Read the model definition and answer for the solid it produces. Units are mm, in the model's axes. Give positions to 0.01 mm unless a question says otherwise; leave off trailing zeros. Order: outer loops, then holes, each group sorted by start corner. A loop starts at its lowest first (then second) coordinate and runs counter-clockwise, first axis right, second up.
Item 1: A cutting plane is placed at A-A (x = -206.5). Write down the section's boundary in (y, z), plus the area to 3 significant figures.
Item 2: A cutting plane is placed at C-C (x = 59.5). Write down the section's boundary in (y, z).
Item 3: A cutting plane is placed at D-D (z = 1.45). State how many separate pieces and enclosed holes the cut face has, plus the area to 3 significant figures.
Item 4: A cutting plane is placed at B-B (y = 66.5). Write down the section's boundary in (x, z).
Item 5: Given pin 1 Ø1.5 at (x, z) = (198.5, 1) entering from -Y; pin 2 Ø0.9 at (y, z) = (233, 2) entering from -X; pin 3 Ø1.5 at (x, z) = (180, 2) entering from +Y, each flat-ended and moving along its own axis, determine where each tip first touches the part or whether it passes through.
Item 6: Find the intervals of material crossed by line 1 along X through (y, z) = (-255, 0.8); line 2 along X through (y, z) = (100, 1.2); line 3 along X through (y, z) = (-108, 1.1), in increasing order.
from build123d import *

# Parameters (mm, degrees)
EXTRUDE_1_DEPTH     = 3
SKETCH_2_R          = 1
CUT_EXTRUDE_1_DEPTH = 3


with BuildPart() as part:
    # 草图1 → 凸台-拉伸1 (new body)
    with BuildSketch(Plane.XY):
        with BuildLine():
            Line((-140, -280), (140, -280))
            ThreePointArc((140, -280), (147.071067812, -277.071067812), (150, -270))
            Line((150, -270), (150, -170))
            ThreePointArc((150, -170), (152.928932188, -162.928932188), (160, -160))
            Line((160, -160), (260, -160))
            ThreePointArc((260, -160), (267.071067812, -157.071067812), (270, -150))
            Line((270, -150), (270, 150))
            ThreePointArc((270, 150), (267.071067812, 157.071067812), (260, 160))
            Line((260, 160), (160, 160))
            ThreePointArc((160, 160), (152.928932188, 162.928932188), (150, 170))
            Line((150, 170), (150, 275))
            ThreePointArc((150, 275), (148.535533906, 278.535533906), (145, 280))
            Line((145, 280), (125, 280))
            ThreePointArc((125, 280), (121.464466094, 281.464466094), (120, 285))
            Line((120, 285), (120, 295))
            ThreePointArc((120, 295), (118.535533906, 298.535533906), (115, 300))
            Line((115, 300), (-115, 300))
            ThreePointArc((-115, 300), (-118.535533906, 298.535533906), (-120, 295))
            Line((-120, 295), (-120, 285))
            ThreePointArc((-120, 285), (-121.464466094, 281.464466094), (-125, 280))
            Line((-125, 280), (-145, 280))
            ThreePointArc((-145, 280), (-148.535533906, 278.535533906), (-150, 275))
            Line((-150, 275), (-150, 170))
            ThreePointArc((-150, 170), (-152.928932188, 162.928932188), (-160, 160))
            Line((-160, 160), (-260, 160))
            ThreePointArc((-260, 160), (-267.071067812, 157.071067812), (-270, 150))
            Line((-270, 150), (-270, -150))
            ThreePointArc((-270, -150), (-267.071067812, -157.071067812), (-260, -160))
            Line((-260, -160), (-160, -160))
            ThreePointArc((-160, -160), (-152.928932188, -162.928932188), (-150, -170))
            Line((-150, -170), (-150, -270))
            ThreePointArc((-150, -270), (-147.071067812, -277.071067812), (-140, -280))
        make_face()
        with BuildLine():
            Line((-90, 240), (90, 240))
            ThreePointArc((90, 240), (97.071067812, 237.071067812), (100, 230))
            Line((100, 230), (100, -230))
            ThreePointArc((100, -230), (97.071067812, -237.071067812), (90, -240))
            Line((90, -240), (-90, -240))
            ThreePointArc((-90, -240), (-97.071067812, -237.071067812), (-100, -230))
            Line((-100, -230), (-100, 230))
            ThreePointArc((-100, 230), (-97.071067812, 237.071067812), (-90, 240))
        make_face(mode=Mode.SUBTRACT)
        with BuildLine():
            Line((-240, 47.5), (-240, 22.5))
            ThreePointArc((-240, 22.5), (-237.071067812, 15.428932188), (-230, 12.5))
            Line((-230, 12.5), (-160, 12.5))
            ThreePointArc((-160, 12.5), (-152.928932188, 15.428932188), (-150, 22.5))
            Line((-150, 22.5), (-150, 47.5))
            ThreePointArc((-150, 47.5), (-152.928932188, 54.571067812), (-160, 57.5))
            Line((-160, 57.5), (-230, 57.5))
            ThreePointArc((-230, 57.5), (-237.071067812, 54.571067812), (-240, 47.5))
        make_face(mode=Mode.SUBTRACT)
        with BuildLine():
            Line((-230, 127.5), (-160, 127.5))
            ThreePointArc((-160, 127.5), (-152.928932188, 124.571067812), (-150, 117.5))
            Line((-150, 117.5), (-150, 92.5))
            ThreePointArc((-150, 92.5), (-152.928932188, 85.428932188), (-160, 82.5))
            Line((-160, 82.5), (-230, 82.5))
            ThreePointArc((-230, 82.5), (-237.071067812, 85.428932188), (-240, 92.5))
            Line((-240, 92.5), (-240, 117.5))
            ThreePointArc((-240, 117.5), (-237.071067812, 124.571067812), (-230, 127.5))
        make_face(mode=Mode.SUBTRACT)
        with BuildLine():
            Line((-240, -22.5), (-240, -47.5))
            ThreePointArc((-240, -47.5), (-237.071067812, -54.571067812), (-230, -57.5))
            Line((-230, -57.5), (-160, -57.5))
            ThreePointArc((-160, -57.5), (-152.928932188, -54.571067812), (-150, -47.5))
            Line((-150, -47.5), (-150, -22.5))
            ThreePointArc((-150, -22.5), (-152.928932188, -15.428932188), (-160, -12.5))
            Line((-160, -12.5), (-230, -12.5))
            ThreePointArc((-230, -12.5), (-237.071067812, -15.428932188), (-240, -22.5))
        make_face(mode=Mode.SUBTRACT)
        with BuildLine():
            Line((-240, -92.5), (-240, -117.5))
            ThreePointArc((-240, -117.5), (-237.071067812, -124.571067812), (-230, -127.5))
            Line((-230, -127.5), (-160, -127.5))
            ThreePointArc((-160, -127.5), (-152.928932188, -124.571067812), (-150, -117.5))
            Line((-150, -117.5), (-150, -92.5))
            ThreePointArc((-150, -92.5), (-152.928932188, -85.428932188), (-160, -82.5))
            Line((-160, -82.5), (-230, -82.5))
            ThreePointArc((-230, -82.5), (-237.071067812, -85.428932188), (-240, -92.5))
        make_face(mode=Mode.SUBTRACT)
        with BuildLine():
            Line((230, -127.5), (160, -127.5))
            ThreePointArc((160, -127.5), (152.928932188, -124.571067812), (150, -117.5))
            Line((150, -117.5), (150, -92.5))
            ThreePointArc((150, -92.5), (152.928932188, -85.428932188), (160, -82.5))
            Line((160, -82.5), (230, -82.5))
            ThreePointArc((230, -82.5), (237.071067812, -85.428932188), (240, -92.5))
            Line((240, -92.5), (240, -117.5))
            ThreePointArc((240, -117.5), (237.071067812, -124.571067812), (230, -127.5))
        make_face(mode=Mode.SUBTRACT)
        with BuildLine():
            Line((230, -57.5), (160, -57.5))
            ThreePointArc((160, -57.5), (152.928932188, -54.571067812), (150, -47.5))
            Line((150, -47.5), (150, -22.5))
            ThreePointArc((150, -22.5), (152.928932188, -15.428932188), (160, -12.5))
            Line((160, -12.5), (230, -12.5))
            ThreePointArc((230, -12.5), (237.071067812, -15.428932188), (240, -22.5))
            Line((240, -22.5), (240, -47.5))
            ThreePointArc((240, -47.5), (237.071067812, -54.571067812), (230, -57.5))
        make_face(mode=Mode.SUBTRACT)
        with BuildLine():
            Line((230, 12.5), (160, 12.5))
            ThreePointArc((160, 12.5), (152.928932188, 15.428932188), (150, 22.5))
            Line((150, 22.5), (150, 47.5))
            ThreePointArc((150, 47.5), (152.928932188, 54.571067812), (160, 57.5))
            Line((160, 57.5), (230, 57.5))
            ThreePointArc((230, 57.5), (237.071067812, 54.571067812), (240, 47.5))
            Line((240, 47.5), (240, 22.5))
            ThreePointArc((240, 22.5), (237.071067812, 15.428932188), (230, 12.5))
        make_face(mode=Mode.SUBTRACT)
        with BuildLine():
            Line((150, 117.5), (150, 92.5))
            ThreePointArc((150, 92.5), (152.928932188, 85.428932188), (160, 82.5))
            Line((160, 82.5), (230, 82.5))
            ThreePointArc((230, 82.5), (237.071067812, 85.428932188), (240, 92.5))
            Line((240, 92.5), (240, 117.5))
            ThreePointArc((240, 117.5), (237.071067812, 124.571067812), (230, 127.5))
            Line((230, 127.5), (160, 127.5))
            ThreePointArc((160, 127.5), (152.928932188, 124.571067812), (150, 117.5))
        make_face(mode=Mode.SUBTRACT)
    extrude(amount=EXTRUDE_1_DEPTH)

    # 草图2 → 切除-拉伸1 (cut)
    with BuildSketch(Plane.XY.offset(3)):
        with Locations((0, 255)):
            Circle(SKETCH_2_R)
        with Locations((70, 255)):
            Circle(SKETCH_2_R)
        with Locations((140, 255)):
            Circle(SKETCH_2_R)
        with Locations((-70, 255)):
            Circle(SKETCH_2_R)
        with Locations((-140, 255)):
            Circle(SKETCH_2_R)
        with Locations((-140, 0)):
            Circle(SKETCH_2_R)
        with Locations((-140, 100)):
            Circle(SKETCH_2_R)
        with Locations((-140, 190)):
            Circle(SKETCH_2_R)
        with Locations((-140, 230)):
            Circle(SKETCH_2_R)
        with Locations((-140, -230)):
            Circle(SKETCH_2_R)
        with Locations((-140, -190)):
            Circle(SKETCH_2_R)
        with Locations((-140, -100)):
            Circle(SKETCH_2_R)
        with Locations((-140, -255)):
            Circle(SKETCH_2_R)
        with Locations((-70, -255)):
            Circle(SKETCH_2_R)
        with Locations((140, -255)):
            Circle(SKETCH_2_R)
        with Locations((70, -255)):
            Circle(SKETCH_2_R)
        with Locations((0, -255)):
            Circle(SKETCH_2_R)
        with Locations((140, -100)):
            Circle(SKETCH_2_R)
        with Locations((140, -190)):
            Circle(SKETCH_2_R)
        with Locations((140, -230)):
            Circle(SKETCH_2_R)
        with Locations((140, 100)):
            Circle(SKETCH_2_R)
        with Locations((140, 0)):
            Circle(SKETCH_2_R)
        with Locations((140, 190)):
            Circle(SKETCH_2_R)
        with Locations((140, 230)):
            Circle(SKETCH_2_R)
    extrude(amount=-CUT_EXTRUDE_1_DEPTH, mode=Mode.SUBTRACT)


solid = part.part
Response values:
1. outline: (-160, 0) - (-127.5, 0) - (-127.5, 3) - (-160, 3) - close; (-82.5, 0) - (-57.5, 0) - (-57.5, 3) - (-82.5, 3) - close; (-12.5, 0) - (12.5, 0) - (12.5, 3) - (-12.5, 3) - close; (57.5, 0) - (82.5, 0) - (82.5, 3) - (57.5, 3) - close; (127.5, 0) - (160, 0) - (160, 3) - (127.5, 3) - close
1. area: 420 mm2
2. outline: (-280, 0) - (-240, 0) - (-240, 3) - (-280, 3) - close; (240, 0) - (300, 0) - (300, 3) - (240, 3) - close
3. separate pieces: 1
3. enclosed holes: 33
3. area: 122,000 mm2
4. outline: (-270, 0) - (-100, 0) - (-100, 3) - (-270, 3) - close; (100, 0) - (270, 0) - (270, 3) - (100, 3) - close
5. pin 1: stops at y = -160
5. pin 2: stops at x = -150
5. pin 3: stops at y = 160
6. line 1: x = -150 to -141, -139 to -71, -69 to -1, 1 to 69, 71 to 139, 141 to 150
6. line 2: x = -270 to -240, -150 to -141, -139 to -100, 100 to 139, 141 to 150, 240 to 270
6. line 3: x = -270 to -240, -150 to -100, 100 to 150, 240 to 270
